Part print with two shaded views. Sizes in mm from the minimum x, y, z corner. A direction names the side the tool comes from. Round coordinates to 2 decimals unless told otherwise and drop trailing zeros. Write each loop counter-clockwise with the first axis right and the second up, starting at its lowest first coordinate (ties: lowest second). Pieces come first, ordered by that corner, then holes. Notation, with made-up numbers: (88.5, 49.5) -> (143.5, 49.5) arc R9 cw to (143.5, 66.5) -> close; hole circle Ø7 at (88.5, 41.5). An arc over 180 degrees is marked (long way). Return JSON: item names as keys, results as strings. Group by question number.
(1) Mould opens along X. For the marked faces 1, 2 and 3 say: +X half, -X half, draft (parallel to the pull), parting line (faces both ways), or undercut.
(2) Drill centre lines: L1, parallel to X at y = 39.25, z = 120; L2, parallel to Z at x = 118, y = 42; L3, parallel to Y at x = 203.5, z = 175. Where is each one in solid material? Low to high. Write a range as from..to.
(3) Saw through at B-B (x = 120). List the corners of the cut face in (y, z), plus the area to 3 significant figures.
(4) Drop flat-ended pins along their axis: pin 1 Ø10 at (x, y) = (151, 21) entering from -Z; pin 2 Ø5 at (x, z) = (47.5, 137.5) entering from -Y; pin 3 Ø5 at (y, z) = (37, 128.5) entering from +X. Give the stop position or say it passes through.
(5) Saw through at D-D (x = 217). List the corners of the cut face in (y, z).
(6) Saw through at A-A (z = 120). List the corners of the cut face in (x, y).
(7) Tool access for the marked faces 4 and 5: list every direction of +Z, -Z, +X, -X, +Y, -Y with a clear straight run to the whole face (end or side of a thin tool).
(8) Saw through at C-C (y = 8.5). List the corners of the cut face in (x, z).
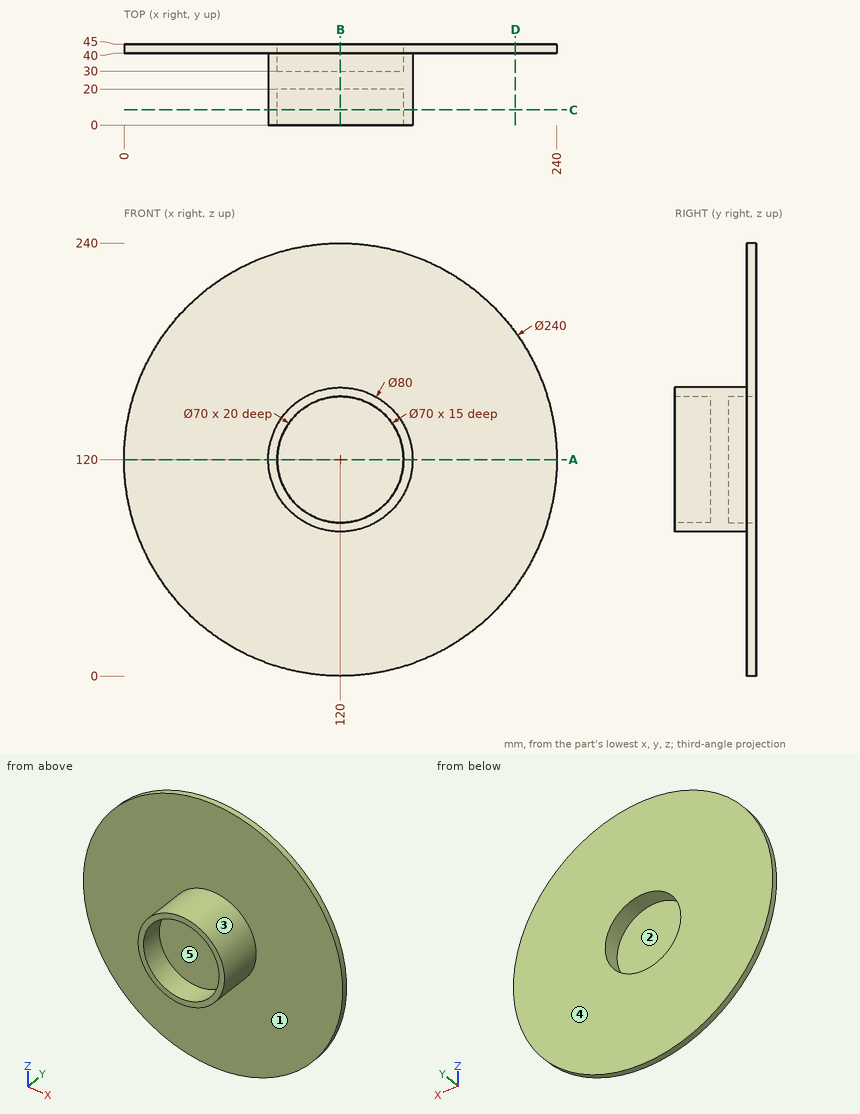
Computed values:
{
 "1": {"face 1": "draft", "face 2": "undercut", "face 3": "parting line"},
 "2": {"L1": "80..85, 155..160", "L2": "0.02..85.06, 154.94..239.98", "L3": "40..45"},
 "3": {"outline": "(0, 80) -> (40, 80) -> (40, 0) -> (45, 0) -> (45, 85) -> (30, 85) -> (30, 155) -> (45, 155) -> (45, 240) -> (40, 240) -> (40, 160) -> (0, 160) -> (0, 155) -> (20, 155) -> (20, 85) -> (0, 85) -> close", "area": "1,950 mm2"},
 "4": {"pin 1": "z = 89.6", "pin 2": "y = 40", "pin 3": "x = 159.55"},
 "5": {"outline": "(40, 49.35) -> (45, 49.35) -> (45, 190.65) -> (40, 190.65) -> close"},
 "6": {"outline": "(0, 40) -> (80, 40) -> (80, 0) -> (85, 0) -> (85, 20) -> (155, 20) -> (155, 0) -> (160, 0) -> (160, 40) -> (240, 40) -> (240, 45) -> (155, 45) -> (155, 30) -> (85, 30) -> (85, 45) -> (0, 45) -> close"},
 "7": {"face 4": "+Z, -Z, +X, -X, +Y", "face 5": "-Y"},
 "8": {"outline": "circle Ø80 at (120, 120); hole circle Ø70 at (120, 120)"}
}
